from build123d import *

# Parameters (mm, degrees)
SKETCH2_R           = 0.75
SKETCH2_R_2         = 1.5
BOSS_EXTRUDE1_DEPTH = 3


with BuildPart() as part:
    # Sketch2 → Boss-Extrude1 (new body)
    with BuildSketch(Plane.XY):
        with BuildLine():
            Line((-9.85, 40.45), (-9.85, 37.45))
            Line((-9.85, 37.45), (-3.75, 37.45))
            Line((-3.75, 37.45), (-3.75, 40.45))
            Line((-3.75, 40.45), (3.75, 40.45))
            Line((3.75, 40.45), (3.75, 37.45))
            Line((3.75, 37.45), (9.85, 37.45))
            Line((9.85, 37.45), (9.85, 40.45))
            Line((9.85, 40.45), (15, 40.45))
            Line((15, 40.45), (15, -25.55))
            ThreePointArc((15, -25.55), (10.63589104, -36.08589104), (0.1, -40.45))
            Line((0.1, -40.45), (-0.1, -40.45))
            ThreePointArc((-0.1, -40.45), (-10.63589104, -36.08589104), (-15, -25.55))
            Line((-15, -25.55), (-15, 40.45))
            Line((-15, 40.45), (-9.85, 40.45))
        make_face()
        with Locations((0, -18.05)):
            Circle(SKETCH2_R, mode=Mode.SUBTRACT)
        with Locations((6.495190528, -21.8)):
            Circle(SKETCH2_R, mode=Mode.SUBTRACT)
        with Locations((6.495190528, -29.3)):
            Circle(SKETCH2_R, mode=Mode.SUBTRACT)
        with Locations((0, -33.05)):
            Circle(SKETCH2_R, mode=Mode.SUBTRACT)
        with Locations((-6.495190528, -29.3)):
            Circle(SKETCH2_R, mode=Mode.SUBTRACT)
        with Locations((-6.495190528, -21.8)):
            Circle(SKETCH2_R, mode=Mode.SUBTRACT)
        with Locations((0, -25.55)):
            Circle(SKETCH2_R_2, mode=Mode.SUBTRACT)
    extrude(amount=BOSS_EXTRUDE1_DEPTH)


solid = part.part
Geometry check sheet. Reference: the model listing, model coordinates, mm. A direction names the side the tool comes from. Round coordinates to 2 decimals unless told otherwise and drop trailing zeros. Loops run counter-clockwise (first coordinate to the right, second up) from the corner with the lowest first, then second, coordinate; pieces in that order, holes last. Notation, with made-up numbers: (29.25, 18) - (61.25, 18) arc R19 ccw to (61.25, 35) - close; hole circle Ø7 at (1.25, 2.5). An arc over 180 degrees is marked (long way). One line per question, with ' | ' between items. Start each with the question number.
1. Scan lines: line 1 (X direction, y = -22, z = 2.8); line 2 (Y direction, x = -6.25, z = 1.75); line 3 (Y direction, x = 12.5, z = 2.5). Record each from-to range of solid material in increasing order. Write a range as [from, to].
2. Cross-section at A-A on y = -18.05. Record the cut outline in (x, z), then the cut area to 3 significant figures.
3. Draft check along Y on faces 3 (the face through (15, 8, 1)), 4 (the face through (12, 40.45, 1)), 5 (the face through (7.188, -22.087, 1.479)), 6 (the face through (-0.098, -32.306, 1.479)). Enter one of: released by +Y, released by -Y, zero draft, split by the parting line, or undercut.
4. Cross-section at D-D on x = -4.5. Record the cut outline in (y, z).
5. Cross-section at C-C on y = -29.3. Record the cut outline in (x, z), then the cut area to 3 significant figures.
6. Depth check by flat-ended pin: pin 1 (1.5 mm diameter, centred on x = 6.5, z = 1.5, fed in from +Y). Enter the tip coordinate at first touch or a pass-through.
7. Cross-section at B-B on z = 2.15. Record the cut outline in (x, y).
8. Tool access check on faces 1 (the face through (6.398, -28.556, 1.479)), 2 (the face through (7, 37.45, 1)). Record the directions out of +Z, -Z, +X, -X, +Y, -Y that give a thin tool (end or side, any length) a straight path to the whole face; none if there is none.
Taken from the geometry:
1) line 1: [-15, -7.22], [-5.77, 5.77], [7.22, 15] | line 2: [-39.12, -30.01], [-28.59, -22.51], [-21.09, 37.45] | line 3: [-33.81, 40.45]
2) outline: (-15, 0) - (-0.75, 0) - (-0.75, 3) - (-15, 3) - close; (0.75, 0) - (15, 0) - (15, 3) - (0.75, 3) - close | area: 85.5 mm²
3) face 3: zero draft | face 4: released by +Y | face 5: undercut | face 6: undercut
4) outline: (-39.79, 0) - (37.45, 0) - (37.45, 3) - (-39.79, 3) - close
5) outline: (-14.52, 0) - (-7.25, 0) - (-7.25, 3) - (-14.52, 3) - close; (-5.75, 0) - (5.75, 0) - (5.75, 3) - (-5.75, 3) - close; (7.25, 0) - (14.52, 0) - (14.52, 3) - (7.25, 3) - close | area: 78.1 mm²
6) pin 1: y = 37.45
7) outline: (-15, -25.55) arc R14.9 ccw to (-0.1, -40.45) - (0.1, -40.45) arc R14.9 ccw to (15, -25.55) - (15, 40.45) - (9.85, 40.45) - (9.85, 37.45) - (3.75, 37.45) - (3.75, 40.45) - (-3.75, 40.45) - (-3.75, 37.45) - (-9.85, 37.45) - (-9.85, 40.45) - (-15, 40.45) - close; hole circle Ø1.5 at (-6.5, -29.3); hole circle Ø1.5 at (-6.5, -21.8); hole circle Ø3 at (0, -25.55); hole circle Ø1.5 at (0, -33.05); hole circle Ø1.5 at (0, -18.05); hole circle Ø1.5 at (6.5, -29.3); hole circle Ø1.5 at (6.5, -21.8)
8) face 1: +Z, -Z | face 2: +Z, -Z, +Y
